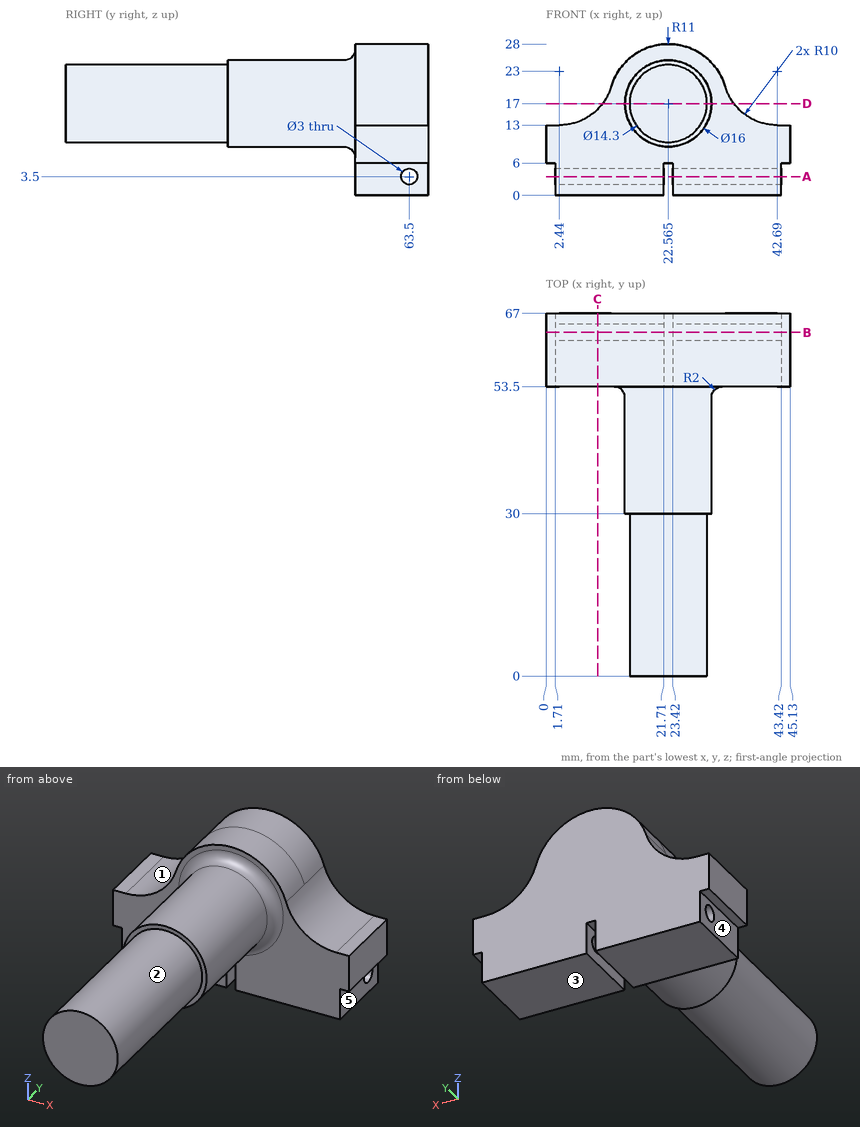
Part print with two shaded views. Sizes in mm from the minimum x, y, z corner. A direction names the side the tool comes from. Coordinates: 2 decimals unless noted, no trailing zeros. Order: outer loops, then holes, each group sorted by start corner. A loop starts at its lowest first (then second) coordinate and runs counter-clockwise, first axis right, second up. Notation, with made-up numbers: M 17,54.25 L 39,54.25 A16 cw 39,67.25 Z; hole C 56,14 d2. An arc over 180 degrees is marked long. Use a Markdown table: item, result.
(1) Cut at D-D on z = 17. Write the cut outline in (x, y) (1 decimal).
A:
| item | result |
|---|---|
| outline | M 10.4,53.5 L 12.6,53.5 A2 cw 14.6,51.5 L 14.6,30 L 15.4,30 L 15.4,0 L 29.7,0 L 29.7,30 L 30.6,30 L 30.6,51.5 A2 cw 32.6,53.5 L 34.7,53.5 L 34.7,67 L 10.4,67 Z |
(2) Flat gauge pins, fed straight in: pin 1 (8.5 mm diameter, centred on x = 33, z = 18.5, fed in from -Y); pin 2 (1.8 mm diameter, centred on y = 60.5, z = 3, fed in from -X); pin 3 (12 mm diameter, centred on y = 30, z = 22.5, fed in from +X) (3 decimals); pin 4 (6 mm diameter, centred on x = 20, y = 37, fed in from +Z). Where does each tip first touch, or does it go through?
A:
| item | result |
|---|---|
| pin 1 | stops at y = 0 |
| pin 2 | stops at x = 1.71 |
| pin 3 | stops at x = 30.565 |
| pin 4 | stops at z = 25 |
(3) Cut at C-C on x = 9.5. Write the cut outline in (y, z), then the cut area to 3 significant figures.
A:
| item | result |
|---|---|
| outline | M 53.5,0 L 67,0 L 67,15.92 L 53.5,15.92 Z; hole C 63.5,3.5 d3 |
| area | 208 mm^2 |
(4) Probe L1, parallel to Y at x = 34.5, z = 3.5; L2, parallel to X at y = 8.5, z = 17 (1 decimal); L3, parallel to Y at x = 33.5, z = 16. List the from-to ranges inside material, lowest first.
A:
| item | result |
|---|---|
| L1 | y = 53.5 to 62, 65 to 67 |
| L2 | x = 15.4 to 29.7 |
| L3 | y = 53.5 to 67 |
(5) Tool access for the marked faces 1, 2, 3, 4 and 5: list every direction of +Z, -Z, +X, -X, +Y, -Y with a clear straight run to the whole face (end or side of a thin tool).
A:
| item | result |
|---|---|
| face 1 | +Z, -X, +Y, -Y |
| face 2 | -Y |
| face 3 | -Z, +X, -X, +Y, -Y |
| face 4 | -Z, -X, +Y, -Y |
| face 5 | -Z, +X, +Y, -Y |
(6) Cut at B-B on y = 63.5. Write the cut outline in (x, z) (1 decimal).
A:
| item | result |
|---|---|
| outline | M 0,6 L 1.7,6 L 1.7,5 L 21.7,5 L 21.7,6 L 23.4,6 L 23.4,5 L 43.4,5 L 43.4,6 L 45.1,6 L 45.1,13 L 42.7,13 A10 cw 33.1,20.1 A11 ccw 12,20.1 A10 cw 2.4,13 L 0,13 Z; M 1.7,0 L 21.7,0 L 21.7,2 L 1.7,2 Z; M 23.4,0 L 43.4,0 L 43.4,2 L 23.4,2 Z |
(7) Cut at A-A on z = 3.5. Write the cut outline in (x, y).
A:
| item | result |
|---|---|
| outline | M 1.71,53.5 L 21.71,53.5 L 21.71,62 L 1.71,62 Z; M 1.71,65 L 21.71,65 L 21.71,67 L 1.71,67 Z; M 23.42,53.5 L 43.42,53.5 L 43.42,62 L 23.42,62 Z; M 23.42,65 L 43.42,65 L 43.42,67 L 23.42,67 Z |
